Study the drawing (mm; zero at the part's minimum x, y, z) and answer. A direction names the side the tool comes from. Round coordinates to 2 decimals unless told otherwise and drop trailing zeros. Write each loop counter-clockwise with the first axis right and the second up, starting at its lowest first coordinate (ties: lowest second). Pieces come first, ordered by that corner, then holes. Notation, with made-up numbers: (-10.5, 87.25) -> (6.5, 87.25) arc R31 ccw to (6.5, 125.25) -> close; hole circle Ø2 at (89, -19). An arc over 180 degrees is marked (long way). Write each question's results on one line, items separated by ' | '. Start each with the question number.
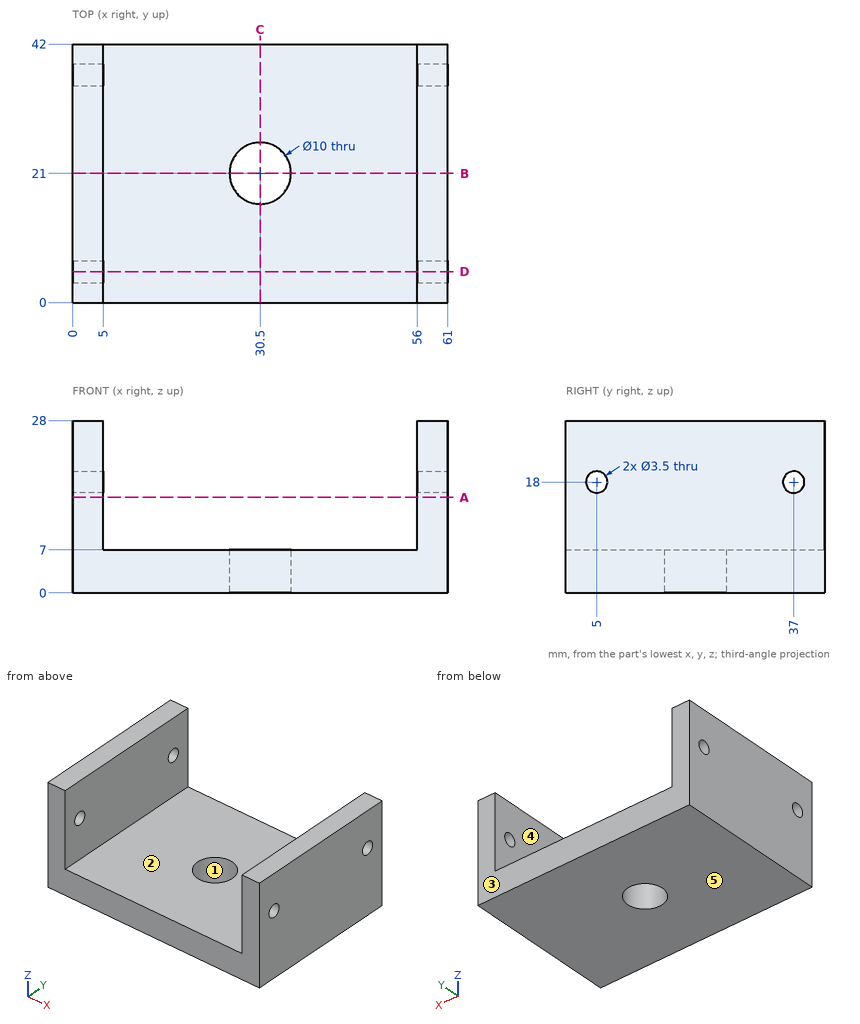
Q1. The part is cut by section C-C, the plane x = 30.5. Write down the section's boundary in (y, z), then the cut area to 3 significant figures.
Q2. The part is cut by section B-B, the plane y = 21. Write down the section's boundary in (x, z).
Q3. The part is cut by section A-A, the plane z = 15.5. Write down the section's boundary in (x, y), then the cut area to 3 significant figures.
Q4. Each of these flat-tipped pins is pushed along its axis until it touches: pin 1 (12 mm diameter, centred on x = 48.5, y = 10, fed in from -Z); pin 2 (12.5 mm diameter, centred on x = 31.5, y = 31.5, fed in from +Z); pin 3 (9 mm diameter, centred on x = 30.5, y = 21, fed in from -Z). Where does it stop, or does it pass through?
Q5. Find the intervals of material crossed by line 1 (X direction, y = 20.5, z = 22.25); line 2 (Z direction, x = 59.1, y = 37); line 3 (Y direction, x = 30.5, z = 2), in increasing order.
Q6. The part is cut by section D-D, the plane y = 5. Write down the section's boundary in (x, z).
Q7. Determine the mould class of the marked faces 1, 2 and 3 for opening direction Y: pulls with the +Y half, pulls with the -Y half, needs draft (parallel to the pull), parting line crosses it, or undercut.
Q8. For the marked faces 4 and 5, determine the directions among +Z, -Z, +X, -X, +Y, -Y from which every point of the face is accessible in a straight line to the end or side of a thin tool.
Answers follow:
1) outline: (0, 0) -> (16, 0) -> (16, 7) -> (0, 7) -> close; (26, 0) -> (42, 0) -> (42, 7) -> (26, 7) -> close | area: 224 mm^2
2) outline: (0, 0) -> (25.5, 0) -> (25.5, 7) -> (5, 7) -> (5, 28) -> (0, 28) -> close; (35.5, 0) -> (61, 0) -> (61, 28) -> (56, 28) -> (56, 7) -> (35.5, 7) -> close
3) outline: (0, 0) -> (5, 0) -> (5, 42) -> (0, 42) -> close; (56, 0) -> (61, 0) -> (61, 42) -> (56, 42) -> close | area: 420 mm^2
4) pin 1: z = 0 | pin 2: z = 7 | pin 3: through
5) line 1: 0 to 5, 56 to 61 | line 2: 0 to 16.25, 19.75 to 28 | line 3: 0 to 16, 26 to 42
6) outline: (0, 0) -> (61, 0) -> (61, 16.25) -> (56, 16.25) -> (56, 7) -> (5, 7) -> (5, 16.25) -> (0, 16.25) -> close; (0, 19.75) -> (5, 19.75) -> (5, 28) -> (0, 28) -> close; (56, 19.75) -> (61, 19.75) -> (61, 28) -> (56, 28) -> close
7) face 1: undercut | face 2: needs draft | face 3: pulls with the +Y half
8) face 4: +Z, +Y, -Y | face 5: -Z, +X, -X, +Y, -Y
